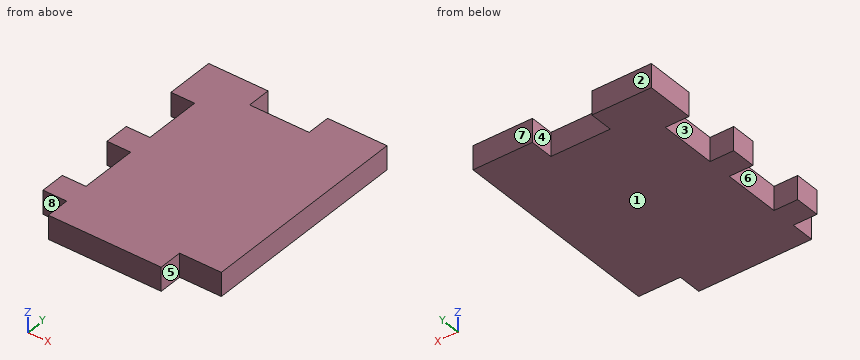
from build123d import *

# Parameters (mm, degrees)
SKETCH1_W           = 40.132
SKETCH1_H           = 53.34
BOSS_EXTRUDE1_DEPTH = 5.334
SKETCH3_W           = 5.334
SKETCH3_H           = 5.334
SKETCH3_W_2         = 9.398
CUT_EXTRUDE1_DEPTH  = 6.334
SKETCH4_W           = 5.334
SKETCH4_H           = 12.954
CUT_EXTRUDE2_DEPTH  = 6.334
SKETCH5_W           = 13.377333334
SKETCH5_H           = 5.334
CUT_EXTRUDE3_DEPTH  = 6.334


with BuildPart() as part:
    # Sketch1 → Boss-Extrude1 (new body)
    with BuildSketch(Plane.XY):
        with Locations((20.066, 26.67)):
            Rectangle(SKETCH1_W, SKETCH1_H)
    extrude(amount=BOSS_EXTRUDE1_DEPTH)

    # Sketch3 → Cut-Extrude1 (cut, through all)
    with BuildSketch(Plane.XY.offset(5.334)):
        with Locations((2.667, 2.667)):
            Rectangle(SKETCH3_W, SKETCH3_H)
        with Locations((35.433, 2.667)):
            Rectangle(SKETCH3_W_2, SKETCH3_H)
    extrude(amount=-CUT_EXTRUDE1_DEPTH, mode=Mode.SUBTRACT)

    # Sketch4 → Cut-Extrude2 (cut, through all)
    with BuildSketch(Plane.XY.offset(5.334)):
        with Locations((2.667, 35.941)):
            Rectangle(SKETCH4_W, SKETCH4_H)
        with Locations((2.667, 17.399)):
            Rectangle(SKETCH4_W, SKETCH4_H)
    extrude(amount=-CUT_EXTRUDE2_DEPTH, mode=Mode.SUBTRACT)

    # Sketch5 → Cut-Extrude3 (cut, through all)
    with BuildSketch(Plane.XY.offset(5.334)):
        with Locations((20.066, 50.673)):
            Rectangle(SKETCH5_W, SKETCH5_H)
    extrude(amount=-CUT_EXTRUDE3_DEPTH, mode=Mode.SUBTRACT)


solid = part.part
Geometry check sheet. Reference: the model listing, model coordinates, mm. Face numbers are marked on the shaded views. A direction names the side the tool comes from. Give positions to 0.01 mm unless a question says otherwise; leave off trailing zeros. Write each loop counter-clockwise with the first axis right and the second up, starting at its lowest first coordinate (ties: lowest second). Pieces come first, ordered by that corner, then holes. Notation, with made-up numbers: (15.25, 44) - (21.25, 44) arc R31 cw to (21.25, 82) - close; hole circle Ø3 at (-7, 7). An arc over 180 degrees is marked (long way). Put each result on its own line as item: value.
1. Sectioned sample at D-D, the plane x = 19.5. Enter the section's corners in (y, z).
Ans:
outline: (0, 0) - (48.01, 0) - (48.01, 5.33) - (0, 5.33) - close
2. Draft check along Y on the marked faces 1, 2 and 3. Enter one of: +Y half, -Y half, draft (parallel to the pull), parting line (faces both ways), or undercut.
Ans:
face 1: draft
face 2: +Y half
face 3: undercut
3. Sectioned sample at B-B, the plane z = 1.5. Enter the section's corners in (x, y).
Ans:
outline: (0, 5.33) - (5.33, 5.33) - (5.33, 0) - (30.73, 0) - (30.73, 5.33) - (40.13, 5.33) - (40.13, 53.34) - (26.75, 53.34) - (26.75, 48.01) - (13.38, 48.01) - (13.38, 53.34) - (0, 53.34) - (0, 42.42) - (5.33, 42.42) - (5.33, 29.46) - (0, 29.46) - (0, 23.88) - (5.33, 23.88) - (5.33, 10.92) - (0, 10.92) - close
4. Go/stop test with flat-tipped pins: pin 1 (2.5 mm diameter, centred on x = 17.5, z = 2.5, fed in from +Y); pin 2 (2.5 mm diameter, centred on y = 16.5, z = 3.5, fed in from -X). Record where each tip stops, or that it passes through.
Ans:
pin 1: stops at y = 48.01
pin 2: stops at x = 5.33
5. Set-up check for the marked faces 4, 5, 6, 7 and 8: record each of +Z, -Z, +X, -X, +Y, -Y from which the full face is reachable in a straight line by a thin tool's end or side.
Ans:
face 4: +Z, -Z, +Y
face 5: +Z, -Z, +X, -Y
face 6: +Z, -Z, -X
face 7: +Z, -Z, +X, -X, +Y
face 8: +Z, -Z, -X, -Y
6. Sectioned sample at C-C, the plane y = 4. Enter the section's corners in (x, z).
Ans:
outline: (5.33, 0) - (30.73, 0) - (30.73, 5.33) - (5.33, 5.33) - close
7. Sectioned sample at A-A, the plane x = 3. Enter the section's corners in (y, z), plus the area to 3 significant figures.
Ans:
outline: (5.33, 0) - (10.92, 0) - (10.92, 5.33) - (5.33, 5.33) - close; (23.88, 0) - (29.46, 0) - (29.46, 5.33) - (23.88, 5.33) - close; (42.42, 0) - (53.34, 0) - (53.34, 5.33) - (42.42, 5.33) - close
area: 118 mm²
8. Thickness scan on line 1 (X direction, y = 36.5, z = 5); line 2 (Y direction, x = 16, z = 3); line 3 (Y direction, x = 37, z = 4.45). Record the ranges inside material, lowest first.
Ans:
line 1: x = 5.33 to 40.13
line 2: y = 0 to 48.01
line 3: y = 5.33 to 53.34
